Verification items for this drawing (mm, ordinates from the low corner). Round coordinates to 2 decimals unless told otherwise and drop trailing zeros. Order: outer loops, then holes, each group sorted by start corner. A loop starts at its lowest first (then second) coordinate and runs counter-clockwise, first axis right, second up. Notation, with made-up numbers: (40.5, 85) -> (55.5, 85) arc R31 cw to (55.5, 119) -> close; hole circle Ø10 at (89.25, 40.25). An arc over 180 degrees is marked (long way). Answer in a Markdown table with one row per item. Add a question column.
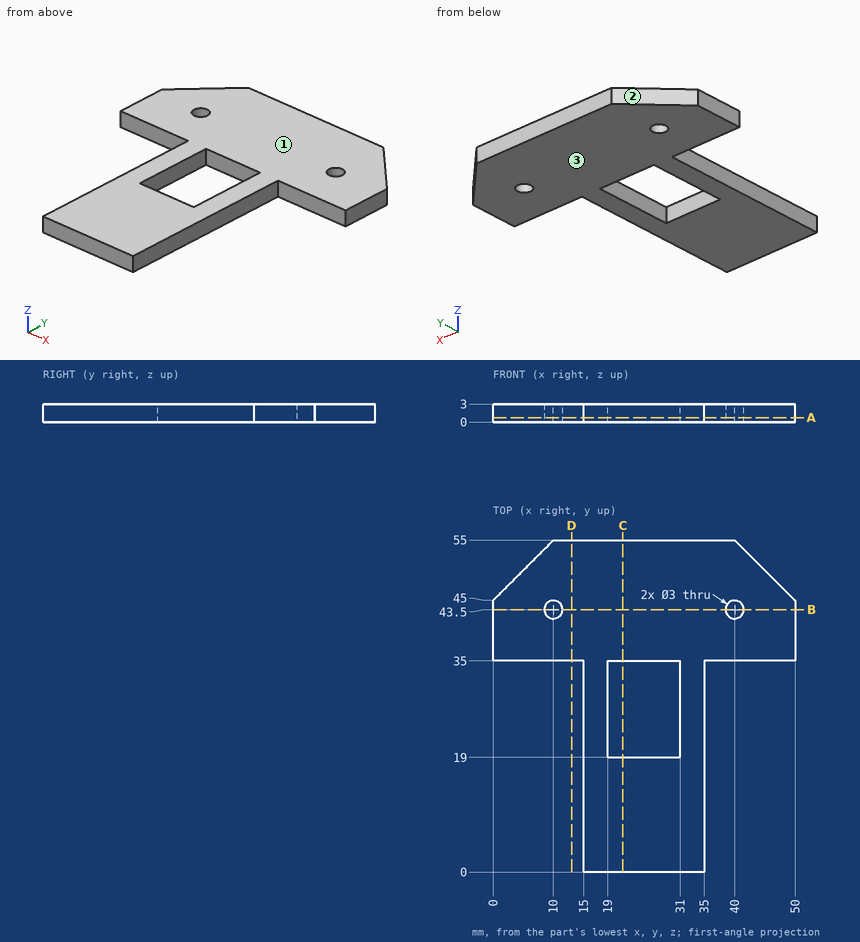
1) Cross-section at C-C, the plane x = 21.5. Record the boundary of the cut face in (y, z).
2) Thickness scan on L1, parallel to Y at x = 40, z = 1.85; L2, parallel to Y at x = 26.5, z = 0.35; L3, parallel to X at y = 24, z = 0.65. Record the ranges inside material, lowest first. Write a range as [from, to].
3) Cross-section at A-A, the plane z = 0.75. Record the boundary of the cut face in (x, y).
4) Cross-section at B-B, the plane y = 43.5. Record the boundary of the cut face in (x, z), and give its area (3 significant figures).
5) Cross-section at D-D, the plane x = 13. Record the boundary of the cut face in (y, z).
6) Depth check by flat-ended pin: P1, Ø1.8, axis at x = 10, y = 43.5, coming from the +Z side; P2, Ø1.5, axis at x = 9.5, z = 2, coming from the -Y side; P3, Ø0.9, axis at y = 11, z = 1, coming from the +X side. Enter the tip coordinate at first touch or a pass-through.
7) Draft check along Z on the marked faces 1, 2 and 3. Enter one of: +Z half, -Z half, draft (parallel to the pull), parting line (faces both ways), or undercut.
Results below:
| question | item | result |
|---|---|---|
| 1 | outline | (0, 0) -> (19, 0) -> (19, 3) -> (0, 3) -> close; (35, 0) -> (55, 0) -> (55, 3) -> (35, 3) -> close |
| 2 | L1 | [35, 42], [45, 55] |
| 2 | L2 | [0, 19], [35, 55] |
| 2 | L3 | [15, 19], [31, 35] |
| 3 | outline | (0, 35) -> (15, 35) -> (15, 0) -> (35, 0) -> (35, 35) -> (50, 35) -> (50, 45) -> (40, 55) -> (10, 55) -> (0, 45) -> close; hole circle Ø3 at (10, 43.5); hole (19, 19) -> (31, 19) -> (31, 35) -> (19, 35) -> close; hole circle Ø3 at (40, 43.5) |
| 4 | outline | (0, 0) -> (8.5, 0) -> (8.5, 3) -> (0, 3) -> close; (11.5, 0) -> (38.5, 0) -> (38.5, 3) -> (11.5, 3) -> close; (41.5, 0) -> (50, 0) -> (50, 3) -> (41.5, 3) -> close |
| 4 | area | 132 mm² |
| 5 | outline | (35, 0) -> (55, 0) -> (55, 3) -> (35, 3) -> close |
| 6 | P1 | through |
| 6 | P2 | y = 35 |
| 6 | P3 | x = 35 |
| 7 | face 1 | +Z half |
| 7 | face 2 | draft |
| 7 | face 3 | -Z half |
